```python
from build123d import *

# Parameters (mm, degrees)
SKETCH1_W           = 120
SKETCH1_H           = 40
BOSS_EXTRUDE1_DEPTH = 25
BOSS_EXTRUDE1_TAPER = 10
SKETCH2_R           = 14
BOSS_EXTRUDE2_DEPTH = 5
SKETCH3_R           = 10
BOSS_EXTRUDE3_DEPTH = 125
SKETCH4_R           = 14
BOSS_EXTRUDE4_DEPTH = 8
SKETCH5_R           = 8
CUT_EXTRUDE1_DEPTH  = 150
FILLET1_R           = 1
SKETCH6_W           = 120
SKETCH6_H           = 40
BOSS_EXTRUDE5_DEPTH = 5


with BuildPart() as part:
    # Sketch1 → Boss-Extrude1 (new body)
    with BuildSketch(Plane(origin=(0, 0, 0), x_dir=(1, 0, 0), z_dir=(0, 1, 0))):
        Rectangle(SKETCH1_W, SKETCH1_H)
    extrude(amount=BOSS_EXTRUDE1_DEPTH, taper=BOSS_EXTRUDE1_TAPER)

    # Sketch2 → Boss-Extrude2 (add)
    with BuildSketch(Plane(origin=(0, 25, 0), x_dir=(1, 0, 0), z_dir=(0, 1, 0))):
        Circle(SKETCH2_R)
    extrude(amount=BOSS_EXTRUDE2_DEPTH)

    # Sketch3 → Boss-Extrude3 (add)
    with BuildSketch(Plane(origin=(0, 30, 0), x_dir=(1, 0, 0), z_dir=(0, 1, 0))):
        Circle(SKETCH3_R)
    extrude(amount=BOSS_EXTRUDE3_DEPTH)

    # Sketch4 → Boss-Extrude4 (add)
    with BuildSketch(Plane(origin=(0, 155, 0), x_dir=(1, 0, 0), z_dir=(0, 1, 0))):
        Circle(SKETCH4_R)
    extrude(amount=BOSS_EXTRUDE4_DEPTH)

    # Sketch5 → Cut-Extrude1 (cut)
    with BuildSketch(Plane(origin=(0, 163, 0), x_dir=(1, 0, 0), z_dir=(0, 1, 0))):
        Circle(SKETCH5_R)
    extrude(amount=-CUT_EXTRUDE1_DEPTH, mode=Mode.SUBTRACT)

    # Fillet1
    fillet1_edges = [part.edges().sort_by_distance(p)[0] for p in [
        (-10, 155, 0),
        (-14, 155, 0),
        (-14, 163, 0),
        (-8, 163, 0),
    ]]
    fillet(fillet1_edges, radius=FILLET1_R)

    # Sketch6 → Boss-Extrude5 (add)
    with BuildSketch(Plane.XZ):
        Rectangle(SKETCH6_W, SKETCH6_H)
    extrude(amount=BOSS_EXTRUDE5_DEPTH)


solid = part.part
```
Verification items for the finished model (mm, model axes). A direction names the side the tool comes from. Round coordinates to 2 decimals unless told otherwise and drop trailing zeros. Order: outer loops, then holes, each group sorted by start corner. A loop starts at its lowest first (then second) coordinate and runs counter-clockwise, first axis right, second up. Notation, with made-up numbers: (-8.75, 0) - (31.25, 0) arc R31 ccw to (31.25, 38) - close; hole circle Ø2 at (73, -7.75). An arc over 180 degrees is marked (long way). Use CSV: the item, a comma, the result in double quotes.
(1) Mould release check, pull along Y, two halves, no side actions. Record for faces 1 (the face through (60, -2, 0)), 2 (the face through (-11, 25, 10)), 3 (the face through (-3, 30, -10)): released by +Y, released by -Y, zero draft, split by the parting line, or undercut.
Entries:
face 1,"zero draft"
face 2,"released by +Y"
face 3,"undercut"
(2) Gauge pin test, flat ends, axial feed: pin 1 Ø6 at (x, y) = (10, 39.5) entering from -Z; pin 2 Ø10 at (y, z) = (19, 12.5) entering from +X; pin 3 Ø5 at (x, y) = (6.5, 88) entering from +Z; pin 4 Ø3 at (y, z) = (39.5, 13) entering from -X. Record the tip position at first contact, or that the pin passes through.
Entries:
pin 1,"z = -7.14"
pin 2,"x = 57.53"
pin 3,"z = 9.17"
pin 4,"through"
(3) Access from +Z, -Z, +X, -X, +Y, -Y to the whole of each face (thin tool, end or side, straight path). Record for faces 4 (the face through (-2.17, 91.13, 9.76)), 5 (the face through (-1, -2, -20)), 6 (the face through (12.932, 27.465, 5.362)).
Entries:
face 4,"none"
face 5,"-Z, +X, -X, +Y, -Y"
face 6,"+Y"
(4) Thickness scan on probe 1 along Z at (x, y) = (0, 81.5); probe 2 along Y at (x, z) = (46, -6). Record the ranges inside material, lowest first. Write a range as from..to.
Entries:
probe 1,"-10..-8, 8..10"
probe 2,"-5..25"
(5) Section check A-A on y = 107. Record the boundary of the cut face in (x, z).
Entries:
outline,"circle Ø20 at (0, 0); hole circle Ø16 at (0, 0)"
